Model file for the job. Use its own axes, mm. Round coordinates to 2 decimals unless told otherwise and drop trailing zeros. Loops run counter-clockwise (first coordinate to the right, second up) from the corner with the lowest first, then second, coordinate; pieces in that order, holes last. Notation, with made-up numbers: M 33,34 L 62,34 A19 ccw 62,64 Z; hole C 3,-16 d7. An arc over 180 degrees is marked long. Answer in a Markdown table with one row per item.
from build123d import *

# Parameters (mm, degrees)
SKETCH1_R           = 17.45
BOSS_EXTRUDE1_DEPTH = 5
SKETCH2_R           = 12.65
BOSS_EXTRUDE2_DEPTH = 6.3
SKETCH3_R           = 12.7
CUT_EXTRUDE1_DEPTH  = 28.14212593
CHAMFER3_SIZE       = 0.25


with BuildPart() as part:
    # Sketch1 → Boss-Extrude1 (new body)
    with BuildSketch(Plane.XY):
        Circle(SKETCH1_R)
    extrude(amount=BOSS_EXTRUDE1_DEPTH)

    # Sketch2 → Boss-Extrude2 (add)
    with BuildSketch(Plane(origin=(0, 0, 0), x_dir=(-1, 0, 0), z_dir=(0, 0, -1))):
        with Locations(Location((0, 0, 0), (0, 0, 180))):
            Circle(SKETCH2_R)
    extrude(amount=BOSS_EXTRUDE2_DEPTH)

    # Sketch3 → Cut-Extrude1 (cut, through all)
    with BuildSketch(Plane.XY.offset(5)):
        Circle(SKETCH3_R)
    extrude(amount=-CUT_EXTRUDE1_DEPTH, mode=Mode.SUBTRACT)

    # Chamfer3
    chamfer3_edges = [part.edges().sort_by_distance(p)[0] for p in [
        (-17.45, 0, 0),
    ]]
    chamfer(chamfer3_edges, length=CHAMFER3_SIZE)


solid = part.part
1. Mould opens along Y. For faces 1 (the flat face through (-1, -13, 0)), 2 (the cylindrical face through (-2.75, -12.4, 2.54)), 3 (the cylindrical face through (-3.783, -17.035, 2.592)) say: +Y half, -Y half, draft (parallel to the pull), parting line (faces both ways), or undercut.
Verdict:
| item | result |
|---|---|
| face 1 | draft |
| face 2 | undercut |
| face 3 | parting line |
2. Pin check, flat tips, straight feed: pin 1 (2 mm diameter, centred on y = 10, z = 2, fed in from +X); pin 2 (1 mm diameter, centred on x = -5.5, y = 10, fed in from -Z); pin 3 (1.5 mm diameter, centred on y = 8.5, z = 0.5, fed in from +X); pin 4 (1 mm diameter, centred on y = -2.5, z = 2.5, fed in from +X) (3 decimals). Stop position of each tip, or through.
Verdict:
| item | result |
|---|---|
| pin 1 | stops at x = 14.95 |
| pin 2 | passes through |
| pin 3 | stops at x = 15.63 |
| pin 4 | stops at x = 17.335 |
3. Saw through at C-C (z = 3.45). Write the cut outline in (x, y), and give its area (3 significant figures).
Verdict:
| item | result |
|---|---|
| outline | C 0,0 d34.9; hole C 0,0 d25.4 |
| area | 450 mm² |
4. Wall check: probe 1 along Y at (x, z) = (0, 2.8); probe 2 along X at (y, z) = (8, 2.6); probe 3 along Y at (x, z) = (-9, 3.55). Give the ranges that are in metal, low to high.
Verdict:
| item | result |
|---|---|
| probe 1 | y = -17.45 to -12.7, 12.7 to 17.45 |
| probe 2 | x = -15.51 to -9.86, 9.86 to 15.51 |
| probe 3 | y = -14.95 to -8.96, 8.96 to 14.95 |
5. Saw through at A-A (x = 0). Write the cut outline in (y, z).
Verdict:
| item | result |
|---|---|
| outline | M -17.45,0.25 L -17.2,0 L -12.7,0 L -12.7,5 L -17.45,5 Z; M 12.7,0 L 17.2,0 L 17.45,0.25 L 17.45,5 L 12.7,5 Z |
